Check sheet for the modelled part. Datum: model origin and axes. Units: mm. Give positions to 0.01 mm unless a question says otherwise; leave off trailing zeros. Order: outer loops, then holes, each group sorted by start corner. A loop starts at its lowest first (then second) coordinate and runs counter-clockwise, first axis right, second up.
Autodesk Inventor part; units mm, degrees
ref_plane "YZ Plane" through (0, 0, 0) normal (1, 0, 0) x (0, 1, 0)
ref_plane "XZ Plane" through (0, 0, 0) normal (0, 1, 0) x (-1, 0, 0)
ref_plane "XY Plane" through (0, 0, 0) normal (0, 0, 1) x (1, 0, 0)
sketch "Szkic1" plane through (0, 0, 0) normal (0, 0, 1) x (1, 0, 0)
  arc A0 (18.7419, 4.0884) -> (15.7419, 7.0884) centre (15.7419, 4.0884) ccw
  line L0 (15.7419, 7.0884) -> (-3.7581, 7.0884)
  arc A1 (-3.7581, 7.0884) -> (-6.7581, 4.0884) centre (-3.7581, 4.0884) ccw
  line L1 (-6.7581, 4.0884) -> (-6.7581, -17.5866)
  arc A2 (-6.7581, -17.5866) -> (-3.7581, -20.5866) centre (-3.7581, -17.5866) ccw
  line L2 (-3.7581, -20.5866) -> (18.7419, -20.5866)
  line L3 (18.7419, -20.5866) -> (18.7419, 4.0884)
  circle A3 centre (12.7419, -14.5866) radius 1.5
  circle A4 centre (12.7419, 1.0884) radius 1.5
  circle A5 centre (-0.7581, 1.0884) radius 1.5
  circle A6 centre (-0.7581, -14.5866) radius 1.5
  point P0 (0, 0)
  point P1 (0, 0)
extrude "Wyciągnięcie proste1" add sketch "Szkic1" along normal blind 4.7
properties part number "3DP_ABS_Induction_Sensor_Mount_Spacer"
1) Material ranges on L1, parallel to Y at x = 11.5, z = 1.7; L2, parallel to Y at x = 13, z = 1.55; L3, parallel to X at y = -15, z = 3.9, recorded low to high.
Recorded:
L1: y = -20.59 to -15.43, -13.75 to 0.25, 1.93 to 7.09
L2: y = -20.59 to -16.06, -13.11 to -0.39, 2.57 to 7.09
L3: x = -6.76 to -2.2, 0.68 to 11.3, 14.18 to 18.74
2) Section check C-C, the plane z = 1.75. Record the cut outline in (x, y).
Recorded:
outline: (-6.76, -17.59) arc R3 ccw to (-3.76, -20.59) - (18.74, -20.59) - (18.74, 4.09) arc R3 ccw to (15.74, 7.09) - (-3.76, 7.09) arc R3 ccw to (-6.76, 4.09) - close; hole circle Ø3 at (-0.76, -14.59); hole circle Ø3 at (-0.76, 1.09); hole circle Ø3 at (12.74, -14.59); hole circle Ø3 at (12.74, 1.09)
3) Section check B-B, the plane y = 0.5. Record the cut outline in (x, z).
Recorded:
outline: (-6.76, 0) - (-2.14, 0) - (-2.14, 4.7) - (-6.76, 4.7) - close; (0.62, 0) - (11.36, 0) - (11.36, 4.7) - (0.62, 4.7) - close; (14.12, 0) - (18.74, 0) - (18.74, 4.7) - (14.12, 4.7) - close
4) Section check A-A, the plane x = -0.25. Record the cut outline in (y, z), then the cut area to 3 significant figures.
Recorded:
outline: (-20.59, 0) - (-16, 0) - (-16, 4.7) - (-20.59, 4.7) - close; (-13.18, 0) - (-0.32, 0) - (-0.32, 4.7) - (-13.18, 4.7) - close; (2.5, 0) - (7.09, 0) - (7.09, 4.7) - (2.5, 4.7) - close
area: 104 mm2
5) Draft check along X on faces 1 (the face through (-5.9, 6.19, 2.32)), 2 (the face through (11.243, -14.653, 2.317)), 3 (the face through (6, 7.088, 2)), 4 (the face through (-1.86, 0.07, 2.32)). Enter one of: +X half, -X half, draft (parallel to the pull), parting line (faces both ways), or undercut.
Recorded:
face 1: -X half
face 2: undercut
face 3: draft
face 4: undercut
6) Depth check by flat-ended pin: pin 1 Ø2.5 at (x, y) = (-0.76, 1.09) entering from -Z. Enter the tip coordinate at first touch or a pass-through.
Recorded:
pin 1: passes through
